from build123d import *

# Parameters (mm, degrees)
SKETCH2_R               = 19.098593171
BOSS_EXTRUDE2_DEPTH     = 20
CUT_EXTRUDE1_START      = -20
CUT_EXTRUDE1_DEPTH      = 20
CIRPATTERN2_COUNT       = 12
SKETCH6_R               = 20.098593171
BOSS_EXTRUDE3_DEPTH     = 2
BOSS_EXTRUDE4_START     = 2
SKETCH7_R               = 20.098593171
BOSS_EXTRUDE4_DEPTH     = 2
CUT_EXTRUDE3_DEPTH      = 38.200899114
CUT_EXTRUDE3_DEPTH_BACK = 38.200899114
SKETCH8_R               = 4.125
SKETCH8_W               = 5.7
SKETCH8_H               = 2.6
CUT_EXTRUDE4_DEPTH      = 46.7367269
CUT_EXTRUDE4_DEPTH_BACK = 46.7367269
SKETCH10_R              = 1.5
CUT_EXTRUDE5_DEPTH      = 10
CUT_EXTRUDE5_DEPTH_BACK = 3
SKETCH11_R              = 3.175
CUT_EXTRUDE6_DEPTH      = 10
CUT_EXTRUDE6_DEPTH_BACK = 3
SKETCH12_R              = 3.15


with BuildPart() as part:
    # Sketch2 → Boss-Extrude2 (new body)
    with BuildSketch(Plane(origin=(0, 0, 0), x_dir=(1, 0, 0), z_dir=(0, 1, 0))):
        with Locations(Location((0, 0, 0), (0, 0, 270))):
            Circle(SKETCH2_R)
    extrude(amount=BOSS_EXTRUDE2_DEPTH)

    # Sketch3 → Cut-Extrude1 (cut)
    with BuildSketch(Plane(origin=(0, 20, 0), x_dir=(1, 0, 0), z_dir=(0, 1, 0)).offset(CUT_EXTRUDE1_START)):
        with BuildLine():
            Line((1.75, 14.598593171), (-1.75, 14.598593171))
            Line((-1.75, 14.598593171), (-2.588214639, 16.901568963))
            ThreePointArc((-2.588214639, 16.901568963), (-3.512123919, 16.734003526), (-4.425441557, 16.515972737))
            Line((-4.425441557, 16.515972737), (-4.943079647, 18.44782439))
            ThreePointArc((-4.943079647, 18.44782439), (0, 19.098593171), (4.943079647, 18.44782439))
            Line((4.943079647, 18.44782439), (4.425441557, 16.515972737))
            ThreePointArc((4.425441557, 16.515972737), (3.512123919, 16.734003526), (2.588214639, 16.901568963))
            Line((2.588214639, 16.901568963), (1.75, 14.598593171))
        make_face()
    cut_extrude1 = extrude(amount=CUT_EXTRUDE1_DEPTH, mode=Mode.SUBTRACT)

    # CirPattern2: Cut-Extrude1 ×12 about axis
    cirpattern2_axis = Axis((0, 0, 0), (0, 1, 0))
    for i in range(1, CIRPATTERN2_COUNT):
        add(cut_extrude1.rotate(cirpattern2_axis, i * 360 / CIRPATTERN2_COUNT), mode=Mode.SUBTRACT)

    # Sketch6 → Boss-Extrude3 (add)
    with BuildSketch(Plane(origin=(0, 20, 0), x_dir=(1, 0, 0), z_dir=(0, 1, 0))):
        with Locations(Location((0, 0, 0), (0, 0, 270))):
            Circle(SKETCH6_R)
    extrude(amount=BOSS_EXTRUDE3_DEPTH)

    # Sketch7 → Boss-Extrude4 (add)
    with BuildSketch(Plane.XZ.offset(BOSS_EXTRUDE4_START)):
        with Locations(Location((0, 0, 0), (0, 0, 90))):
            Circle(SKETCH7_R)
    extrude(amount=-BOSS_EXTRUDE4_DEPTH)

    # Sketch8 → Cut-Extrude3 (cut, two sides: drawn at the far end of the back side and taken through both)
    with BuildSketch(Plane.XZ.offset(2).offset(-CUT_EXTRUDE3_DEPTH_BACK)):
        with Locations(Location((0, 0, 0), (0, 0, 270))):
            Circle(SKETCH8_R)
        with Locations((0, 9.425)):
            Rectangle(SKETCH8_W, SKETCH8_H)
        with Locations((0, -9.425)):
            Rectangle(SKETCH8_W, SKETCH8_H)
    extrude(amount=CUT_EXTRUDE3_DEPTH + CUT_EXTRUDE3_DEPTH_BACK, mode=Mode.SUBTRACT)

    # Sketch10 → Cut-Extrude4 (cut, two sides: drawn at the far end of the back side and taken through both)
    with BuildSketch(Plane(origin=(0, 0, -14.598593171), x_dir=(-1, 0, 0), z_dir=(0, 0, -1)).offset(-CUT_EXTRUDE4_DEPTH_BACK)):
        with Locations((0, 10)):
            Circle(SKETCH10_R)
    extrude(amount=CUT_EXTRUDE4_DEPTH + CUT_EXTRUDE4_DEPTH_BACK, mode=Mode.SUBTRACT)

    # Sketch11 → Cut-Extrude5 (cut, two sides: drawn at the far end of the back side and taken through both)
    with BuildSketch(Plane(origin=(0, 0, -14.598593171), x_dir=(-1, 0, 0), z_dir=(0, 0, -1)).offset(-CUT_EXTRUDE5_DEPTH_BACK)):
        with Locations(Location((0, 10, 0), (0, 0, 144.605728901))):
            Circle(SKETCH11_R)
    extrude(amount=CUT_EXTRUDE5_DEPTH + CUT_EXTRUDE5_DEPTH_BACK, mode=Mode.SUBTRACT)

    # Sketch12 → Cut-Extrude6 (cut, two sides: drawn at the far end of the back side and taken through both)
    with BuildSketch(Plane.XY.offset(14.598593171).offset(-CUT_EXTRUDE6_DEPTH_BACK)):
        with Locations(Location((0, 10, 0), (0, 0, 145.250854713))):
            Circle(SKETCH12_R)
    extrude(amount=CUT_EXTRUDE6_DEPTH + CUT_EXTRUDE6_DEPTH_BACK, mode=Mode.SUBTRACT)


solid = part.part
Could you check a few things on this model? Use its own coordinates, in mm. A direction names the side the tool comes from. Round coordinates to 2 decimals unless told otherwise and drop trailing zeros. Write each loop counter-clockwise with the first axis right and the second up, starting at its lowest first coordinate (ties: lowest second). Pieces come first, ordered by that corner, then holes. Notation, with made-up numbers: (44, -19.5) - (91, -19.5) arc R34 ccw to (91, 14.5) - close; hole circle Ø4 at (-3, 43.25). An arc over 180 degrees is marked (long way). Use a Markdown table: item, result.
Q1. For pin 1 (1 mm diameter, centred on y = 9, z = 0, fed in from +X); pin 2 (6 mm diameter, centred on y = 13.5, z = 9, fed in from +X); pin 3 (1.9 mm diameter, centred on x = 1, y = 10, fed in from -Z), each with a flat end and sliding along its axis, tell me the tip position at first contact or that it passes through.
Output values:
| item | result |
|---|---|
| pin 1 | x = 14.6 |
| pin 2 | x = 16.01 |
| pin 3 | z = -11.6 |
Q2. I want a section at A-A (y = 20.5). List the corners of the cut face in (x, z) for me (3 decimals), plus the area to 3 significant figures.
Output values:
| item | result |
|---|---|
| outline | circle Ø40.197 at (0, 0); hole circle Ø8.25 at (0, 0); hole (-2.85, -10.725) - (2.85, -10.725) - (2.85, -8.125) - (-2.85, -8.125) - close; hole (-2.85, 8.125) - (2.85, 8.125) - (2.85, 10.725) - (-2.85, 10.725) - close |
| area | 1,190 mm2 |
Q3. Please list where these lines run through material, in increasing order: L1, parallel to Y at x = 0, z = 12; L2, parallel to Y at x = 6, z = -14; L3, parallel to Z at x = 1, y = 14.75 (3 decimals).
Output values:
| item | result |
|---|---|
| L1 | -2 to 6.85, 13.15 to 22 |
| L2 | -2 to 0, 20 to 22 |
| L3 | -14.599 to -10.725, -8.125 to -4.002, 4.002 to 8.125, 10.725 to 14.599 |
Q4. I want a section at D-D (z = 7). List the corners of the cut face in (x, y) for me, plus the area to 3 significant figures.
Output values:
| item | result |
|---|---|
| outline | (-18.84, -2) - (18.84, -2) - (18.84, 0) - (12.82, 0) - (12.82, 20) - (18.84, 20) - (18.84, 22) - (-18.84, 22) - (-18.84, 20) - (-12.82, 20) - (-12.82, 0) - (-18.84, 0) - close; hole circle Ø3 at (0, 10) |
| area | 656 mm2 |
Q5. I want a section at C-C (x = 0). Count the separate pieces of the cut face and the enclosed holes in it, plus the area to 3 significant figures.
Output values:
| item | result |
|---|---|
| separate pieces | 8 |
| enclosed holes | 0 |
| area | 355 mm2 |
Q6. For faces 5 (the flat face through (2.175, 4.023, -15.766)), 6 (the flat face through (6, 9.86, 14.74)), 7 (the flat face through (9.74, 9.86, 12.544)), 8 (the flat face through (-15.766, 9.86, -2.175)), which set-ups out of +Z, -Z, +X, -X, +Y, -Y let a thin tool reach every point of the face, with its end or its side?
Output values:
| item | result |
|---|---|
| face 5 | -Z |
| face 6 | +X |
| face 7 | +Z |
| face 8 | -X |
Q7. I want a section at B-B (z = 0). List the corners of the cut face in (x, y) for me (3 decimals).
Output values:
| item | result |
|---|---|
| outline | (-20.099, -2) - (-4.125, -2) - (-4.125, 22) - (-20.099, 22) - (-20.099, 20) - (-14.599, 20) - (-14.599, 0) - (-20.099, 0) - close; (4.125, -2) - (20.099, -2) - (20.099, 0) - (14.599, 0) - (14.599, 20) - (20.099, 20) - (20.099, 22) - (4.125, 22) - close |
Q8. Thinking about a two-plate mould opening in X: for faces 1 (the flat face through (0, 22, -5)), 2 (the flat face through (-2, 10, 11.599)), 3 (the cylindrical face through (0.325, 8.536, 11.168)), 4 (the flat face through (5.994, 9.86, -14.708)), which applies, released by +X, released by -X, zero draft, split by the parting line, or undercut?
Output values:
| item | result |
|---|---|
| face 1 | zero draft |
| face 2 | undercut |
| face 3 | undercut |
| face 4 | released by +X |
